Geometry: final body of the model. Coordinates: model frame, mm. Face numbers are marked on the shaded views. A direction names the side the tool comes from. Give positions to 0.01 mm unless a question says otherwise; leave off trailing zeros. Write each loop counter-clockwise with the first axis right and the second up, starting at its lowest first coordinate (ties: lowest second). Pieces come first, ordered by that corner, then holes. Notation, with made-up numbers: (52, 83) -> (82, 83) arc R29 cw to (82, 122) -> close; hole circle Ø7 at (52.25, -22). An arc over 180 degrees is marked (long way). Answer as a JSON object with one key per item and string values. Group by question number.
(1) Set-up query: the marked faces 4, 5 and 6. Return all of +Z, -Z, +X, -X, +Y, -Y with unobstructed straight access to the full face (end or side cutting, diameter ignored); none if empty.
(2) Contact query for flat-ended pins moving along their axis: pin 1 Ø12 at (x, z) = (2, 1.5) entering from -Y; pin 2 Ø16.5 at (y, z) = (0, 0) entering from +X; pin 3 Ø3 at (x, y) = (-10.5, 1.5) entering from -Z; pin 4 Ø1.5 at (x, y) = (-7, 10.5) entering from +Z. Output: stop coordinate, or through.
(3) Section query C-C on x = 10. Output: boundary loops of the cut face in (y, z) (1 decimal), plus the area to 3 significant figures.
(4) Draft query along Z for the marked faces 1, 2 and 3. Return one class per face: +Z half, -Z half, draft (parallel to the pull), parting line (faces both ways), or undercut.
(5) Section query A-A on z = 0. Output: boundary loops of the cut face in (x, y).
(6) Section query D-D on x = -5. Output: boundary loops of the cut face in (y, z).
(7) Material intervals for probe 1 along Z at (x, y) = (-9.5, 0); probe 2 along Z at (x, y) = (-2, 0); probe 3 along Y at (x, z) = (-12, 8), sorted ascending.
from build123d import *

# Parameters (mm, degrees)
F0_R     = 38.1
F0_R_2   = 14.2875
F1_DEPTH = 19.05
F0_R_3   = 6.35
F2_DEPTH = 6.35
F3_R     = 6.35


with BuildPart() as f1:
    # F0 (on Right) → F1 (new body, symmetric)
    with BuildSketch(Plane.YZ):
        Circle(F0_R)
        Circle(F0_R_2, mode=Mode.SUBTRACT)
    extrude(amount=F1_DEPTH, both=True)

    # F0 (on Right) → F2 (join, symmetric)
    with BuildSketch(Plane.YZ):
        Circle(F0_R_2)
        Circle(F0_R_3, mode=Mode.SUBTRACT)
    extrude(amount=F2_DEPTH, both=True)

    # F3
    f3_edges = [f1.edges().sort_by_distance(p)[0] for p in [
        (-19.05, -14.2875, 0),
        (19.05, -14.2875, 0),
    ]]
    fillet(f3_edges, radius=F3_R)


solid = f1.part
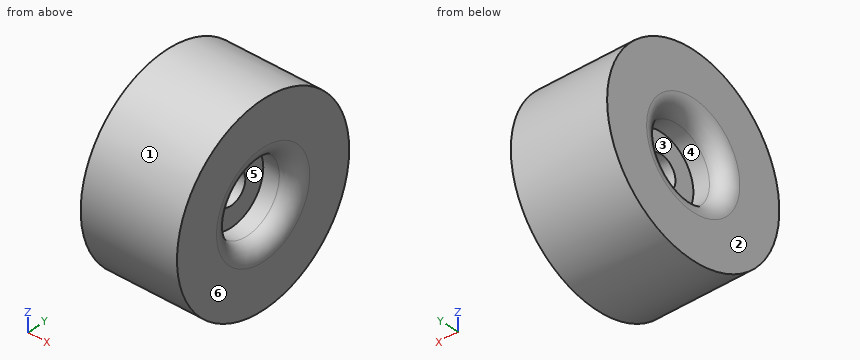
Answer list:
{
 "1": {"face 4": "-X", "face 5": "+X", "face 6": "+Z, -Z, +X, +Y, -Y"},
 "2": {"pin 1": "y = -38.1", "pin 2": "x = 6.35", "pin 3": "z = -38.1", "pin 4": "z = 36.83"},
 "3": {"outline": "circle Ø76.2 at (0, 0); hole circle Ø28.6 at (0, 0)", "area": "3,920 mm2"},
 "4": {"face 1": "parting line", "face 2": "draft", "face 3": "undercut"},
 "5": {"outline": "(-19.05, -38.1) -> (19.05, -38.1) -> (19.05, -20.64) arc R6.35 ccw to (12.7, -14.29) -> (6.35, -14.29) -> (6.35, -6.35) -> (-6.35, -6.35) -> (-6.35, -14.29) -> (-12.7, -14.29) arc R6.35 ccw to (-19.05, -20.64) -> close; (-19.05, 20.64) arc R6.35 ccw to (-12.7, 14.29) -> (-6.35, 14.29) -> (-6.35, 6.35) -> (6.35, 6.35) -> (6.35, 14.29) -> (12.7, 14.29) arc R6.35 ccw to (19.05, 20.64) -> (19.05, 38.1) -> (-19.05, 38.1) -> close"},
 "6": {"outline": "circle Ø76.2 at (0, 0); hole circle Ø12.7 at (0, 0)"},
 "7": {"probe 1": "-38.1 to -14.29, 14.29 to 38.1", "probe 2": "-38.1 to -6.35, 6.35 to 38.1", "probe 3": "-37.25 to -11.84, 11.84 to 37.25"}
}
